Model file for the job. Use its own axes, mm. Face numbers are marked on the shaded views. A direction names the side the tool comes from. Round coordinates to 2 decimals unless told otherwise and drop trailing zeros. Loops run counter-clockwise (first coordinate to the right, second up) from the corner with the lowest first, then second, coordinate; pieces in that order, holes last. Notation, with made-up numbers: M 64.25,-19.5 L 102.25,-19.5 A23 ccw 102.25,12.5 Z; hole C 70,45 d5. An arc over 180 degrees is marked long. Answer in a Markdown table with one row per item.
from build123d import *

# Parameters (mm, degrees)
F0_R          = 14.2875
F0_R_2        = 12.7
F2_DEPTH      = 50.8
F3_R          = 26.9875
F3_R_2        = 14.2875
F4_DEPTH      = 63.5
F4_DEPTH_BACK = 12.7
F5_SIZE       = 7.62


with BuildPart() as f2:
    # F0 (on Top) → F2 (new body)
    with BuildSketch(Plane.XY):
        Circle(F0_R)
        Circle(F0_R_2, mode=Mode.SUBTRACT)
    extrude(amount=F2_DEPTH)

    # F3 (on face) → F4 (join, two sides)
    with BuildSketch(Plane.XY) as f4_sk:
        Circle(F3_R)
        Circle(F3_R_2, mode=Mode.SUBTRACT)
    extrude(amount=F4_DEPTH)
    extrude(f4_sk.sketch, amount=-F4_DEPTH_BACK)

    # F5
    f5_edges = [f2.edges().sort_by_distance(p)[0] for p in [
        (-26.9875, 0, 63.5),
        (-26.9875, 0, -12.7),
    ]]
    chamfer(f5_edges, length=F5_SIZE)


solid = f2.part
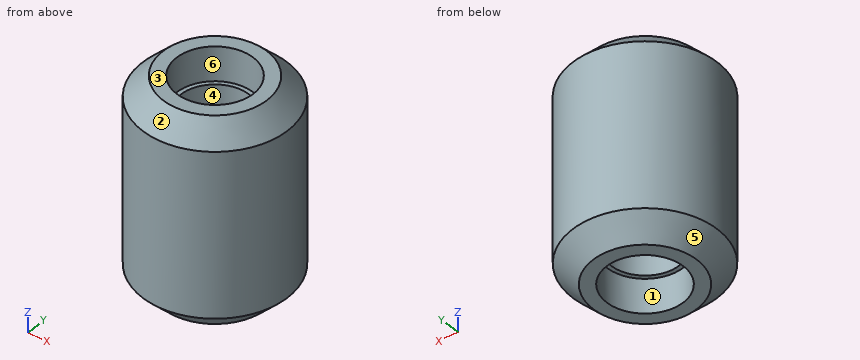
1. Mould opens along X. For the marked faces 1, 2, 3 and 4 say: +X half, -X half, draft (parallel to the pull), parting line (faces both ways), or undercut.
Verdict:
| item | result |
|---|---|
| face 1 | undercut |
| face 2 | parting line |
| face 3 | draft |
| face 4 | undercut |
2. Tool access for the marked faces 5 and 6: list every direction of +Z, -Z, +X, -X, +Y, -Y with a clear straight run to the whole face (end or side of a thin tool).
Verdict:
| item | result |
|---|---|
| face 5 | -Z |
| face 6 | +Z |
3. Pin check, flat tips, straight feed: pin 1 (3 mm diameter, centred on x = -18, z = 27.5, fed in from -Y); pin 2 (2 mm diameter, centred on x = -2, z = 49.5, fed in from +Y); pin 3 (10 mm diameter, centred on y = 20.5, z = 6.5, fed in from +X). Stop position of each tip, or through.
Verdict:
| item | result |
|---|---|
| pin 1 | stops at y = -21.36 |
| pin 2 | stops at y = 26.97 |
| pin 3 | stops at x = 22.09 |
4. Wall check: probe 1 along Y at (x, z) = (0, 27); probe 2 along Y at (x, z) = (0, -3); probe 3 along Z at (x, y) = (-13, 1). Give the ranges that are in metal, low to high.
Verdict:
| item | result |
|---|---|
| probe 1 | y = -26.99 to -12.7, 12.7 to 26.99 |
| probe 2 | y = -26.99 to -14.29, 14.29 to 26.99 |
| probe 3 | z = 0 to 50.8 |
5. Saw through at C-C (z = -1). Write the cut outline in (x, y) (1 decimal).
Verdict:
| item | result |
|---|---|
| outline | C 0,0 d54; hole C 0,0 d28.6 |
6. Saw through at A-A (y = 0). Write the cut outline in (x, z).
Verdict:
| item | result |
|---|---|
| outline | M -26.99,-5.08 L -19.37,-12.7 L -14.29,-12.7 L -14.29,0 L -12.7,0 L -12.7,50.8 L -14.29,50.8 L -14.29,63.5 L -19.37,63.5 L -26.99,55.88 Z; M 12.7,0 L 14.29,0 L 14.29,-12.7 L 19.37,-12.7 L 26.99,-5.08 L 26.99,55.88 L 19.37,63.5 L 14.29,63.5 L 14.29,50.8 L 12.7,50.8 Z |
